Geometry check sheet. Reference: the model listing, model coordinates, mm. Face numbers are marked on the shaded views. A direction names the side the tool comes from. Round coordinates to 2 decimals unless told otherwise and drop trailing zeros. Write each loop counter-clockwise with the first axis right and the second up, starting at its lowest first coordinate (ties: lowest second). Pieces come first, ordered by that corner, then holes. Notation, with made-up numbers: M 5,36 L 22,36 A29 ccw 22,61 Z; hole C 87,56.25 d11. An arc over 180 degrees is marked long. One line per item, written item: value. Start each with the question number.
1. Section check B-B (y = 5). Record the boundary of the cut face in (x, z).
2. Scan lines: probe 1 along Y at (x, z) = (-5, 1.6); probe 2 along Y at (x, z) = (-10, 1.6); probe 3 along Y at (x, z) = (-17, 3.35). Record each from-to range of solid material in increasing order. Write a range as [from, to].
3. Access from +Z, -Z, +X, -X, +Y, -Y to the whole of each face (thin tool, end or side, straight path). Record for the marked faces 5 and 6.
4. Release check for a two-part mould opening along Y. For the marked faces 1, 2, 3 and 4 record: pulls with the +Y half, pulls with the -Y half, needs draft (parallel to the pull), parting line crosses it, or undercut.
5. Section check C-C (x = -5). Record the boundary of the cut face in (y, z).
6. Section check D-D (z = 4.3). Record the boundary of the cut face in (x, y).
7. Section check A-A (x = -21.5). Record the boundary of the cut face in (y, z), and give its area (3 significant figures).
8. Depth check by flat-ended pin: P1, Ø4, axis at x = -25.5, y = 47, coming from the +Z side; P2, Ø1.5, axis at y = 24, z = 1.5, coming from the +X side; P3, Ø4, axis at x = -32.5, y = 8.5, coming from the -Z side. Enter the tip coordinate at first touch or a pass-through.
from build123d import *

# Parameters (mm, degrees)
SKETCH_1_R      = 1.7
EXTRUDE_1_DEPTH = 5
FILLET_1_R      = 3
CHAMFER_1_SIZE  = 3


with BuildPart() as part:
    # 草图1 → 凸台-拉伸1 (new body)
    with BuildSketch(Plane.XY):
        Polygon((0, 0), (-55, 0), (-55, 56.2), (0, 56.2), (0, 49.2), (-45, 49.2), (-45, 10), (0, 10), align=None)
        with Locations((-10, 5)):
            Circle(SKETCH_1_R, mode=Mode.SUBTRACT)
        with Locations((-28, 5)):
            Circle(SKETCH_1_R, mode=Mode.SUBTRACT)
        with Locations((-5, 53.2)):
            Circle(SKETCH_1_R, mode=Mode.SUBTRACT)
        with Locations((-34.46, 53.2)):
            Circle(SKETCH_1_R, mode=Mode.SUBTRACT)
    extrude(amount=EXTRUDE_1_DEPTH)

    # 圆角1
    fillet_1_edges = [part.edges().sort_by_distance(p)[0] for p in [
        (0, 0, 2.5),
        (-55, 0, 2.5),
        (-55, 56.2, 2.5),
        (0, 10, 2.5),
    ]]
    fillet(fillet_1_edges, radius=FILLET_1_R)

    # 倒角1
    chamfer_1_edges = [part.edges().sort_by_distance(p)[0] for p in [
        (-45, 49.2, 2.5),
        (-45, 10, 2.5),
    ]]
    chamfer(chamfer_1_edges, length=CHAMFER_1_SIZE)


solid = part.part
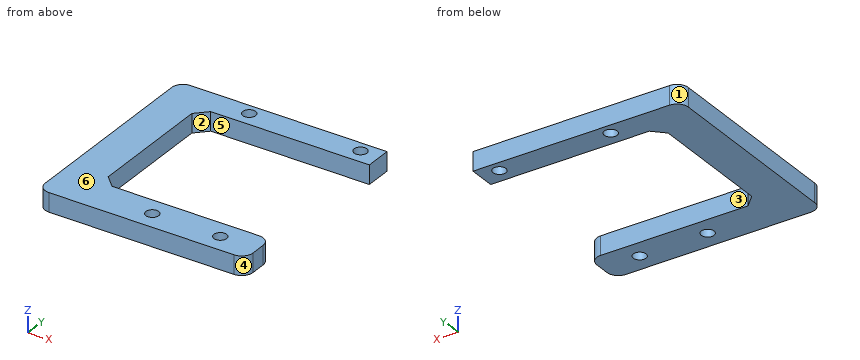
Result sheet:
1. outline: M -55,0 L -29.7,0 L -29.7,5 L -55,5 Z; M -26.3,0 L -11.7,0 L -11.7,5 L -26.3,5 Z; M -8.3,0 L 0,0 L 0,5 L -8.3,5 Z
2. probe 1: y = [0, 10], [49.2, 51.5], [54.9, 56.2]
2. probe 2: y = [0, 3.3], [6.7, 10], [49.2, 56.2]
2. probe 3: y = [0, 10], [49.2, 56.2]
3. face 5: +Z, -Z, +X
3. face 6: +Z, +X, -X, +Y, -Y
4. face 1: pulls with the +Y half
4. face 2: undercut
4. face 3: undercut
4. face 4: pulls with the -Y half
5. outline: M 0,0 L 10,0 L 10,5 L 0,5 Z; M 49.2,0 L 51.5,0 L 51.5,5 L 49.2,5 Z; M 54.9,0 L 56.2,0 L 56.2,5 L 54.9,5 Z
6. outline: M -55,3 A3 ccw -52,0 L -3,0 A3 ccw 0,3 L 0,7 A3 ccw -3,10 L -42,10 L -45,13 L -45,46.2 L -42,49.2 L 0,49.2 L 0,56.2 L -52,56.2 A3 ccw -55,53.2 Z; hole C -34.46,53.2 d3.4; hole C -28,5 d3.4; hole C -10,5 d3.4; hole C -5,53.2 d3.4
7. outline: M 0,0 L 10,0 L 10,5 L 0,5 Z; M 49.2,0 L 56.2,0 L 56.2,5 L 49.2,5 Z
7. area: 85.0 mm2
8. P1: passes through
8. P2: stops at x = -45
8. P3: stops at z = 0
